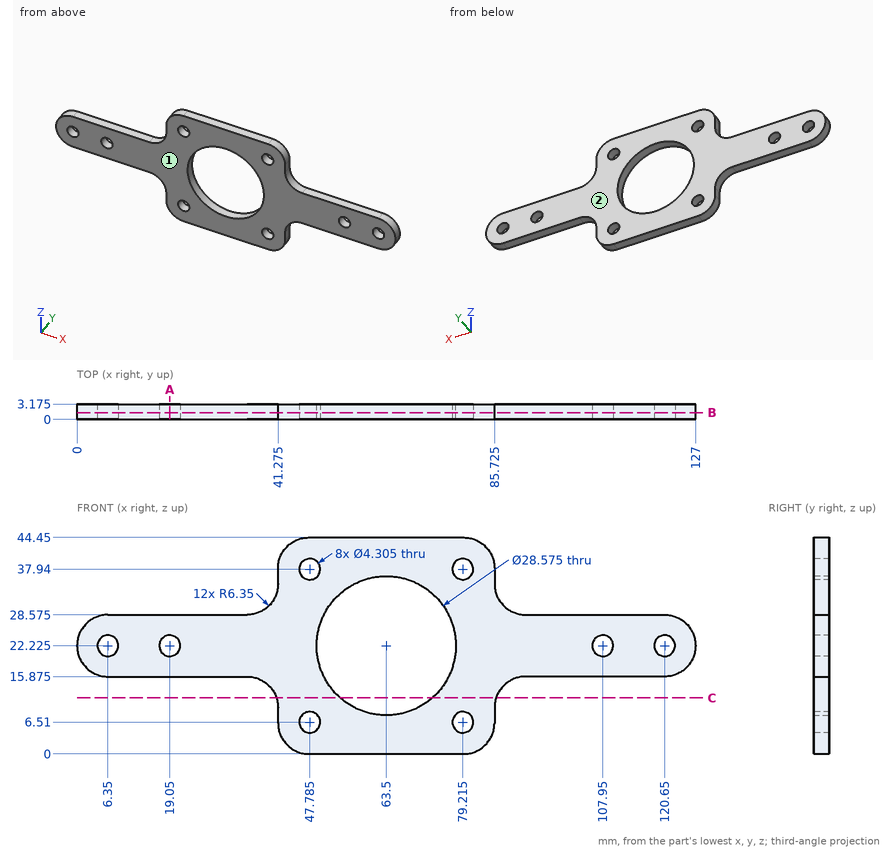
The drawing under review shows one solid part. Ordinate dimensions are in mm from its lowest x, y, z. Give positions to 0.01 mm unless a question says otherwise; leave off trailing zeros. Write each loop counter-clockwise with the first axis right and the second up, starting at its lowest first coordinate (ties: lowest second). Pieces come first, ordered by that corner, then holes. Notation, with made-up numbers: (75, -5) - (122, -5) arc R28 ccw to (122, 29) - close; hole circle Ø11 at (-1.5, 8.25). An arc over 180 degrees is marked (long way). Answer in a Markdown table with one row per item. Add a question column.
1. Wall thickness on line 1 along Z through (x, y) = (79, 0.4); line 2 along X through (y, z) = (2.2, 22) (1 decimal); line 3 along Z through (x, y) = (107.95, 1.25) (1 decimal): over which ranges is each line inside the solid? List them lowest first. Write a range as [from, to].
2. We need section B-B on y = 1.4. State how many separate pieces and enclosed holes the cut face has, then the cut area to 3 significant figures.
3. We need section A-A on x = 19.05. Write out the cut boundary in (y, z) (1 decimal).
4. We need section C-C on z = 11.5. Write out the cut boundary in (x, y) (1 decimal).
5. Draft analysis for pull direction Y (two halves, no side actions). For the marked faces 1 and 2, state which applies: +Y half, -Y half, draft (parallel to the pull), parting line (faces both ways), or undercut.
6. Insertion check: P1, Ø4, axis at x = 47.78, z = 37.94, coming from the +Y side; P2, Ø1.6, axis at x = 24.5, y = 1.5, coming from the +Z side (3 decimals); P3, Ø1, axis at y = 1.5, z = 7, coming from the +X side (3 decimals). Each pin has a flat end and moves straight along its axis. Give the tip position at first contact, or say it passes through.
Ans:
| question | item | result |
|---|---|---|
| 1 | line 1 | z = [0, 4.37], [8.65, 35.8], [40.08, 44.45] |
| 1 | line 2 | x = [0, 4.2], [8.5, 16.9], [21.2, 49.2], [77.8, 105.8], [110.1, 118.5], [122.8, 127] |
| 1 | line 3 | z = [15.9, 20.1], [24.4, 28.6] |
| 2 | separate pieces | 1 |
| 2 | enclosed holes | 9 |
| 2 | area | 2,230 mm^2 |
| 3 | outline | (0, 15.9) - (3.2, 15.9) - (3.2, 20.1) - (0, 20.1) - close; (0, 24.4) - (3.2, 24.4) - (3.2, 28.6) - (0, 28.6) - close |
| 4 | outline | (41, 0) - (54.1, 0) - (54.1, 3.2) - (41, 3.2) - close; (72.9, 0) - (86, 0) - (86, 3.2) - (72.9, 3.2) - close |
| 5 | face 1 | -Y half |
| 5 | face 2 | +Y half |
| 6 | P1 | passes through |
| 6 | P2 | stops at z = 28.575 |
| 6 | P3 | stops at x = 85.725 |
